Read the model definition and answer for the solid it produces. Units are mm, in the model's axes. Give positions to 0.01 mm unless a question says otherwise; leave off trailing zeros. Order: outer loops, then holes, each group sorted by start corner. A loop starts at its lowest first (then second) coordinate and runs counter-clockwise, first axis right, second up. Notation, with made-up numbers: M 52,-4.5 L 72,-4.5 A31 cw 72,25.5 Z; hole C -29,-38.75 d3. An arc over 180 degrees is marked long. One line per item, written item: value. Start each with the question number.
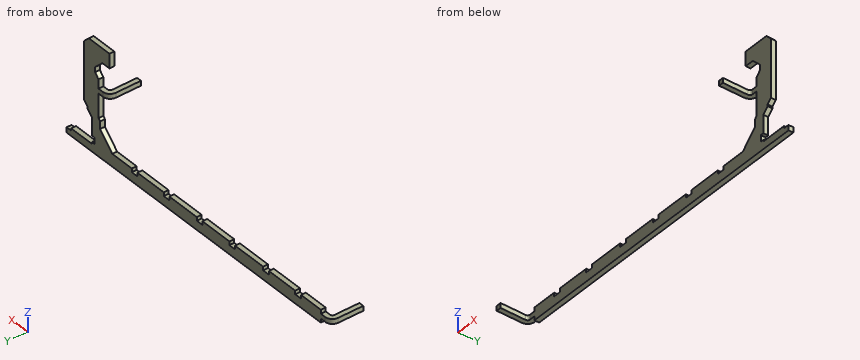
from build123d import *

# Parameters (mm, degrees)
SKETCH1_W           = 2.25
SKETCH1_H           = 2
BOSS_EXTRUDE1_DEPTH = 2
SKETCH12_W          = 3
SKETCH12_H          = 2.15
SKETCH12_W_2        = 2.99999908
SKETCH12_W_3        = 2.89999928
SKETCH12_W_4        = 2
SKETCH12_H_2        = 2.69999968
SKETCH12_H_3        = 2
CUT_EXTRUDE1_DEPTH  = 10
EDGE_FLANGE1_DEPTH  = 2
EDGE_FLANGE2_DEPTH  = 2


# Sheet-metal steps are written as plain solids
with BuildPart() as part:
    # Sketch1 → Boss-Extrude1 (new body)
    with BuildSketch(Plane(origin=(0, 0, 0), x_dir=(1, 0, 0), z_dir=(0, 1, 0))):
        with Locations((47.911990623, -24.171897133)):
            Rectangle(SKETCH1_W, SKETCH1_H)
        with Locations((-67.346417942, -0.378635375)):
            Rectangle(SKETCH1_W, SKETCH1_H)
        Polygon((49.036990623, -28.925083001), (49.036990623, -13.225081484), (48.236992223, -12.425083084), (48.236992223, -9.325081664), (41.890545314, -2.978634755), (-54.913007717, -2.978634755), (-66.221417942, -2.978634755), (-66.221417942, 2.221364005), (-54.913007717, 2.221364005), (65.536992183, 2.221364005), (65.536992183, -0.878636415), (52.536992783, -0.878636415), (52.536992783, -11.632189325), (54.736991299, -13.832187841), (54.736993839, -14.532188981), (56.436992603, -16.232187745), (56.436992603, -40.185676156), (54.062239478, -42.560429281), (43.336991863, -42.560429281), (43.336991863, -36.616688347), (47.052491322, -36.616688347), (50.836992103, -32.832187565), (50.836992103, -30.725081941), align=None)
    extrude(amount=BOSS_EXTRUDE1_DEPTH)

    # Sketch12 → Cut-Extrude1 (cut)
    with BuildSketch(Plane(origin=(0, 2, 0), x_dir=(1, 0, 0), z_dir=(0, 1, 0))):
        with Locations((-54.413012042, -2.553635995)):
            Rectangle(SKETCH12_W, SKETCH12_H)
        with Locations((-37.813011762, -2.553635995)):
            Rectangle(SKETCH12_W_2, SKETCH12_H)
        with Locations((-20.263011302, -2.553635995)):
            Rectangle(SKETCH12_W_3, SKETCH12_H)
        with Locations((-3.363012082, -2.553635995)):
            Rectangle(SKETCH12_W_3, SKETCH12_H)
        with Locations((13.736989278, -2.553635995)):
            Rectangle(SKETCH12_W_3, SKETCH12_H)
        with Locations((30.336989098, -2.553635995)):
            Rectangle(SKETCH12_W_3, SKETCH12_H)
        with Locations((52.186988038, -2.878639758)):
            Rectangle(SKETCH12_W_4, SKETCH12_H_2)
        with Locations((64.636989078, -0.978635995)):
            Rectangle(SKETCH12_W_3, SKETCH12_H_3)
    extrude(amount=-CUT_EXTRUDE1_DEPTH, mode=Mode.SUBTRACT)

    # Edge-Flange1 section (across the edge) → Edge-Flange1 (add)
    with BuildSketch(Plane(origin=(-69.471417942, 0, 1.378635375), x_dir=(1, 0, 0), z_dir=(0, 0, -1))):
        with BuildLine():
            Line((-2, 1), (-2, 11.4))
            Line((-2, 11.4), (0, 11.4))
            Line((0, 11.4), (0, 1))
            ThreePointArc((0, 1), (0.292893219, 0.292893219), (1, 0))
            Line((1, 0), (1, -2))
            ThreePointArc((1, -2), (-1.121320344, -1.121320344), (-2, 1))
        make_face()
    extrude(amount=EDGE_FLANGE1_DEPTH)

    # Edge-Flange2 section (across the edge) → Edge-Flange2 (add)
    with BuildSketch(Plane(origin=(45.786990623, 0, 25.171897133), x_dir=(1, 0, 0), z_dir=(0, 0, -1))):
        with BuildLine():
            Line((-2, 1), (-2, 11.4))
            Line((-2, 11.4), (0, 11.4))
            Line((0, 11.4), (0, 1))
            ThreePointArc((0, 1), (0.292893219, 0.292893219), (1, 0))
            Line((1, 0), (1, -2))
            ThreePointArc((1, -2), (-1.121320344, -1.121320344), (-2, 1))
        make_face()
    extrude(amount=EDGE_FLANGE2_DEPTH)


solid = part.part
Q1. Find section A-A, the plane y = -6. Give the vertices of the cut face in (x, z).
Q2. Consider probe 1 along X at (y, z) = (1.5, 10); probe 2 along Z at (x, y) = (-16.5, 1); probe 3 along Y at (x, z) = (54, 22). Determine where each line is inside the solid, lowest interval first.
Q3. Each of these flat-tipped pins is pushed along its axis until it touches: pin 1 (2.5 mm diameter, centred on x = 45.5, y = -2.5, fed in from -Z); pin 2 (1 mm diameter, centred on y = 0.5, z = 7.5, fed in from +X); pin 3 (2 mm diameter, centred on y = -8, z = 24.5, fed in from -X). Where does it stop, or does it pass through?
Q4. Find section C-C, the plane x = -45. Give the vertices of the cut face in (y, z), then the cut area to 3 significant figures.
Q5. Find section B-B, the plane x = -20. Give the vertices of the cut face in (y, z), then the cut area to 3 significant figures.
Evaluation:
1. outline: M -71.47,-0.62 L -69.47,-0.62 L -69.47,1.38 L -71.47,1.38 Z; M 43.79,23.17 L 45.79,23.17 L 45.79,25.17 L 43.79,25.17 Z
2. probe 1: 48.24 to 52.54
2. probe 2: -2.22 to 2.98
2. probe 3: 0 to 2
3. pin 1: z = 23.17
3. pin 2: x = 52.54
3. pin 3: x = 43.79
4. outline: M 0,-2.22 L 2,-2.22 L 2,2.98 L 0,2.98 Z
4. area: 10.4 mm2
5. outline: M 0,-2.22 L 2,-2.22 L 2,1.48 L 0,1.48 Z
5. area: 7.40 mm2
